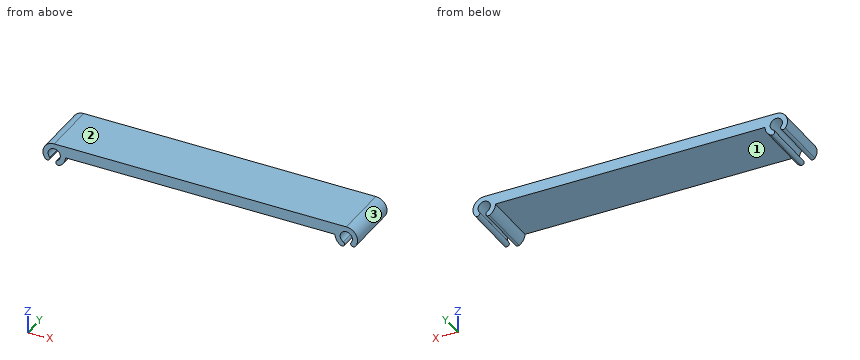
from build123d import *

# Parameters (mm, degrees)
RESSALTO_EXTRUS_O1_DEPTH = 30


with BuildPart() as part:
    # Esboço1 → Ressalto-extrusão1 (new body)
    with BuildSketch(Plane(origin=(0, 0, 0), x_dir=(1, 0, 0), z_dir=(0, 1, 0))):
        with BuildLine():
            Line((-72, 0), (72, 0))
            ThreePointArc((72, 0), (72.85009345, 3.078711179), (75.159487509, 5.285024956))
            ThreePointArc((75.159487509, 5.285024956), (77.004661638, 4.729916917), (76.449553599, 2.884742789))
            ThreePointArc((76.449553599, 2.884742789), (77.536782743, -3.242075689), (80.296246294, 2.335139815))
            ThreePointArc((80.296246294, 2.335139815), (81.096189798, 3.978813584), (82.863892701, 3.513196237))
            ThreePointArc((82.863892701, 3.513196237), (83.342245662, -2.731375348), (78, -6))
            Line((78, -6), (-78, -6))
            ThreePointArc((-78, -6), (-83.342245662, -2.731375348), (-82.863892701, 3.513196237))
            ThreePointArc((-82.863892701, 3.513196237), (-81.096189798, 3.978813584), (-80.296246294, 2.335139815))
            ThreePointArc((-80.296246294, 2.335139815), (-77.536782743, -3.242075689), (-76.449553599, 2.884742789))
            ThreePointArc((-76.449553599, 2.884742789), (-77.004661638, 4.729916917), (-75.159487509, 5.285024956))
            ThreePointArc((-75.159487509, 5.285024956), (-72.85009345, 3.078711179), (-72, 0))
        make_face()
    extrude(amount=RESSALTO_EXTRUS_O1_DEPTH)


solid = part.part
The model under review builds one solid part; all positions refer to its coordinate system, in mm. Face numbers are marked on the shaded views. Give positions to 0.01 mm unless a question says otherwise; leave off trailing zeros. Write each loop counter-clockwise with the first axis right and the second up, starting at its lowest first coordinate (ties: lowest second). Pieces come first, ordered by that corner, then holes.
1. For P1, Ø2, axis at x = 35.5, z = 0.5, coming from the -Y side; P2, Ø2, axis at x = -60.5, y = 17.5, coming from the -Z side; P3, Ø1.5, axis at y = 13.5, z = -1, coming from the +X side; P4, Ø1.5, axis at y = 11.5, z = 4.5, coming from the +X side, all flat-tipped, find the tip position at first contact; note any pin that passes through.
2. Draft analysis for pull direction X (two halves, no side actions). For the marked faces 1, 2 and 3, state which applies: +X half, -X half, draft (parallel to the pull), parting line (faces both ways), or undercut.
3. Add section B-B, the plane x = 29.5. Write out the cut boundary in (y, z).
4. Wall thickness on L1, parallel to X at y = 7.75, z = -0.25; L2, parallel to X at y = 27.5, z = 0.5; L3, parallel to X at y = 4, z = 2.25: over which ranges is each line inside the solid? List them lowest first.
Worked answers:
1. P1: stops at y = 0
1. P2: stops at z = 0
1. P3: stops at x = 83.99
1. P4: stops at x = 82.68
2. face 1: undercut
2. face 2: draft
2. face 3: +X half
3. outline: (0, 0) - (30, 0) - (30, 6) - (0, 6) - close
4. L1: x = -83.99 to -81.27, -74.73 to -72.01, 72.01 to 74.73, 81.27 to 83.99
4. L2: x = -83.98 to -81.24, -74.76 to 74.76, 81.24 to 83.98
4. L3: x = -83.56 to -80.38, -75.62 to 75.62, 80.38 to 83.56
